Check sheet for the modelled part. Datum: model origin and axes. Units: mm. A direction names the side the tool comes from. Give positions to 0.01 mm unless a question says otherwise; leave off trailing zeros. Answer as CSV lines item,"result". Start each with the question number.
(1) Release check for a two-part mould opening along X. For faces 6 (the face through (158.69, 51.66, 1.57)), 7 (the face through (63.409, -110.038, 1.565)), 8 (the face through (40, 3, 0)) record: pulls with the +X half, pulls with the -X half, needs draft (parallel to the pull), parting line crosses it, or undercut.
(2) Gauge pin test, flat ends, axial feed: pin 1 Ø3.5 at (x, y) = (0, 38.1) entering from -Z; pin 2 Ø1.5 at (y, z) = (68.5, 2.5) entering from -X. Record the tip position at first contact, or that the pin passes through.
(3) Section check A-A on z = 1.65. State how many separate pieces and enclosed holes the cut face has, plus the area to 3 significant figures.
(4) Material ranges on line 1 (Y direction, x = 0, z = 1.35); line 2 (X direction, y = 64.5, z = 2.4); line 3 (Y direction, x = 14, z = 1.95), recorded low to high. Write a range as from..to.
(5) Access from +Z, -Z, +X, -X, +Y, -Y to the whole of each face (thin tool, end or side, straight path). Record for faces 1 (the face through (182.08, -73.84, 1.57)), 2 (the face through (-110.507, -104.496, 1.565)), 3 (the face through (-145.75, 43.454, 1.565)), 4 (the face through (-182.82, -89.75, 1.57)), 5 (the face through (-124.087, 111.603, 1.565)).
from build123d import *

# Parameters (mm, degrees)
SKETCH1_R            = 127
BOSS_EXTRUDE1_DEPTH  = 3.175
BOSS_EXTRUDE2_DEPTH  = 3.175
CIRPATTERN2_COUNT    = 6
CUT_EXTRUDE1_DEPTH   = 281.459484309
M5_CLEARANCE_HOLE1_D = 5.5
CIRPATTERN3_COUNT    = 6


with BuildPart() as part:
    # Sketch1 → Boss-Extrude1 (new body)
    with BuildSketch(Plane.XY):
        Circle(SKETCH1_R)
    extrude(amount=BOSS_EXTRUDE1_DEPTH)

    # Sketch6 → Boss-Extrude2 (add)
    with BuildSketch(Plane(origin=(0, 0, 0), x_dir=(-1, 0, 0), z_dir=(0, 0, -1))):
        with BuildLine():
            Line((-49.339907198, 69.180942427), (-133.608436136, 117.833400293))
            ThreePointArc((-133.608436136, 117.833400293), (-155.29169035, 120.688054866), (-172.642612049, 107.37422438))
            Line((-172.642612049, 107.37422438), (-193.280112049, 71.629025839))
            Line((-193.280112049, 71.629025839), (-84.264907198, 8.689067972))
            Line((-84.264907198, 8.689067972), (-49.339907198, 69.180942427))
        make_face()
    boss_extrude2 = extrude(amount=-BOSS_EXTRUDE2_DEPTH)

    # CirPattern2: Boss-Extrude2 ×6 about axis
    cirpattern2_axis = Axis((0, 0, 0), (0, 0, 1))
    for i in range(1, CIRPATTERN2_COUNT):
        add(boss_extrude2.rotate(cirpattern2_axis, i * 360 / CIRPATTERN2_COUNT))

    # Sketch7 → Cut-Extrude1 (cut, through all)
    with BuildSketch(Plane.XY.offset(3.175)):
        Polygon((7.332348419, 0), (3.666174209, 6.35), (-3.666174209, 6.35), (-7.332348419, 0), (-3.666174209, -6.35), (3.666174209, -6.35), align=None)
    extrude(amount=-CUT_EXTRUDE1_DEPTH, mode=Mode.SUBTRACT)

    # M5 Clearance Hole1 (through all)
    with Locations(Plane(origin=(0, 0, 0), x_dir=(-1, 0, 0), z_dir=(0, 0, -1))):
        with Locations((-62.218505846, 54.252742145), (-78.093505846, 26.756435575), (-81.866135768, 10.60369343), (-109.211644375, 33.723978604), (-83.811644375, 77.718069116), (-50.116135768, 65.59630657), (-32.995567884, 19.05), (-10.998522628, 6.35)):
            m5_clearance_hole1 = Hole(M5_CLEARANCE_HOLE1_D / 2)

    # CirPattern3: M5 Clearance Hole1 ×6 about axis
    cirpattern3_axis = Axis((0, 0, 0), (0, 0, 1))
    for i in range(1, CIRPATTERN3_COUNT):
        add(m5_clearance_hole1.rotate(cirpattern3_axis, i * 360 / CIRPATTERN3_COUNT), mode=Mode.SUBTRACT)


solid = part.part
Working result:
1,face 6,"pulls with the +X half"
1,face 7,"undercut"
1,face 8,"needs draft"
2,pin 1,"passes through"
2,pin 2,"stops at x = -180.36"
3,separate pieces,"1"
3,enclosed holes,"49"
3,area,"81,000 mm^2"
4,line 1,"y = -203.2..-40.85, -35.35..-15.45, -9.95..-6.35, 6.35..9.95, 15.45..35.35, 40.85..203.2"
4,line 2,"x = -177.5..-52.64, -47.59..47.59, 52.64..180.93"
4,line 3,"y = -202.24..-83.02, -79..79, 83.02..203.2"
5,face 1,"+Z, -Z, +X"
5,face 2,"+Z, -Z, -Y"
5,face 3,"+Z, -Z, -X"
5,face 4,"+Z, -Z, -X, -Y"
5,face 5,"+Z, -Z, +Y"
